Geometry: final body of the model. Coordinates: model frame, mm. Face numbers are marked on the shaded views. A direction names the side the tool comes from. Give positions to 0.01 mm unless a question says otherwise; leave off trailing zeros. Write each loop counter-clockwise with the first axis right and the second up, starting at its lowest first coordinate (ties: lowest second). Pieces come first, ordered by that corner, then holes. Notation, with made-up numbers: (51, -38) -> (58, -38) arc R18 ccw to (58, -18) -> close; hole circle Ø8 at (48, 73). An arc over 180 degrees is marked (long way). Answer as a JSON object with one key per item and string values.
Autodesk Inventor part; units mm, degrees
ref_plane "YZ Plane" through (0, 0, 0) normal (1, 0, 0) x (0, 1, 0)
ref_plane "XZ Plane" through (0, 0, 0) normal (0, 1, 0) x (-1, 0, 0)
ref_plane "XY Plane" through (0, 0, 0) normal (0, 0, 1) x (1, 0, 0)
sketch "Szkic1" plane through (0, 0, 0) normal (0, 1, 0) x (-1, 0, 0)
  circle A0 centre (0, 0) radius 16
  circle A1 centre (5.5, 0) radius 5.5
  circle A2 centre (5.5, 0) radius 4
  dimension "d1" = 11
  dimension "d0" = 32
  dimension "d2" = 8
extrude "Wyciągnięcie proste1" add sketch "Szkic1" along normal blind 40 contours A0
extrude "Wyciągnięcie proste2" add sketch "Szkic1" along normal blind 42 contours A1
extrude "Wyciągnięcie proste3" add sketch "Szkic1" along normal blind 60 contours A2
properties part number "silnik"
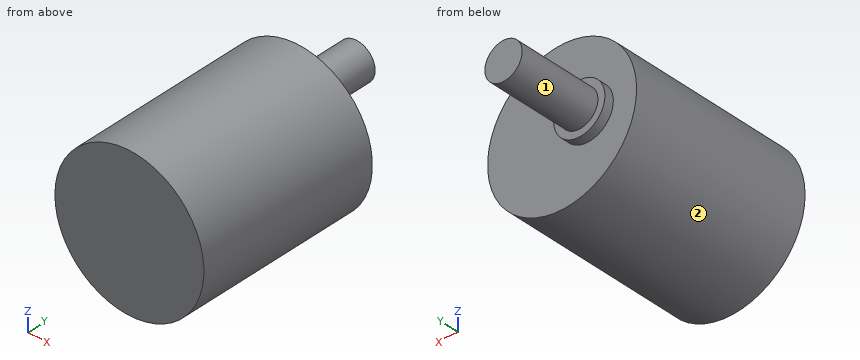
Q1. Material intervals for L1, parallel to Y at x = 3, z = 4.5; L2, parallel to Z at x = -10, y = 21.5; L3, parallel to Z at x = 5.5, y = 34, sorted ascending. Write a range as from..to.
Values:
{"L1": "0..40", "L2": "-12.49..12.49", "L3": "-15.02..15.02"}
Q2. Set-up query: the marked faces 1 and 2. Return all of +Z, -Z, +X, -X, +Y, -Y with unobstructed straight access to the full face (end or side cutting, diameter ignored); none if empty.
Values:
{"face 1": "+Y", "face 2": "+Y, -Y"}
Q3. Cut plane A-A (z = 0). Return the cut outline in (x, y), and give its area (3 significant figures).
Values:
{"outline": "(-16, 0) -> (16, 0) -> (16, 40) -> (0, 40) -> (0, 42) -> (-1.5, 42) -> (-1.5, 60) -> (-9.5, 60) -> (-9.5, 42) -> (-11, 42) -> (-11, 40) -> (-16, 40) -> close", "area": "1,450 mm²"}
Q4. Cut plane B-B (x = -5.5). Return the cut outline in (y, z), and give its area (3 significant figures).
Values:
{"outline": "(0, -15.02) -> (40, -15.02) -> (40, -5.5) -> (42, -5.5) -> (42, -4) -> (60, -4) -> (60, 4) -> (42, 4) -> (42, 5.5) -> (40, 5.5) -> (40, 15.02) -> (0, 15.02) -> close", "area": "1,370 mm²"}
Q5. First-contact query: P1, Ø1, axis at x = -0.5, y = 41, coming from the -Z side; P2, Ø1, axis at y = 25.5, z = -8.5, coming from the +X side; P3, Ø10, axis at y = 51.5, z = 8.5, coming from the -X side. Flat tips, straight axial feed; report the tip coordinate or a pass-through.
Values:
{"P1": "z = -3.16", "P2": "x = 13.86", "P3": "x = -7.44"}
Q6. Cut plane D-D (x = 7.5). Return the cut outline in (y, z), and give its area (3 significant figures).
Values:
{"outline": "(0, -14.13) -> (40, -14.13) -> (40, 14.13) -> (0, 14.13) -> close", "area": "1,130 mm²"}
Q7. Cut plane C-C (y = 15.5). Return the cut outline in (x, z), and give its area (3 significant figures).
Values:
{"outline": "circle Ø32 at (0, 0)", "area": "804 mm²"}
